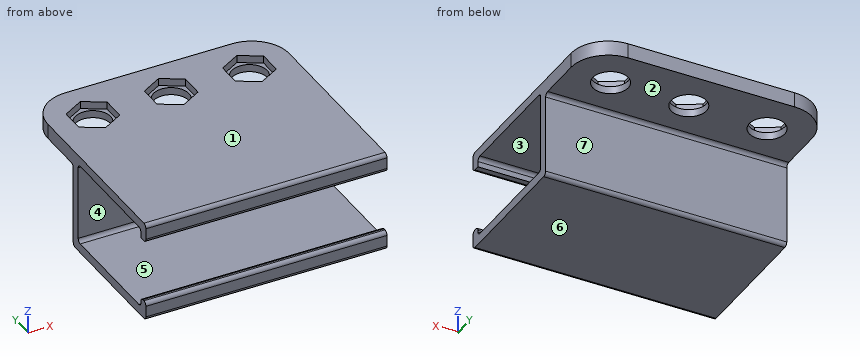
```python
from build123d import *

# Parameters (mm, degrees)
SKETCH_W     = 64.701706
SKETCH_H     = 22.701706
PAD_DEPTH    = 2
SKETCH001_W  = 64.701706
SKETCH001_H  = 22.701706
SKETCH001_R  = 4.75
PAD001_DEPTH = 2
PAD002_DEPTH = 64.701706
FILLET_R     = 10
FILLET001_R  = 1


with BuildPart() as part:
    # Sketch → Pad (new body)
    with BuildSketch(Plane.XY):
        Rectangle(SKETCH_W, SKETCH_H)
        Polygon((0, 6.350853), (-5.5, 3.175426), (-5.5, -3.175426), (0, -6.350853), (5.5, -3.175426), (5.5, 3.175426), align=None, mode=Mode.SUBTRACT)
        Polygon((-21, 6.350853), (-26.5, 3.175426), (-26.5, -3.175426), (-21, -6.350853), (-15.5, -3.175426), (-15.5, 3.175426), align=None, mode=Mode.SUBTRACT)
        Polygon((21, 6.350853), (15.5, 3.175426), (15.5, -3.175426), (21, -6.350853), (26.5, -3.175426), (26.5, 3.175426), align=None, mode=Mode.SUBTRACT)
    extrude(amount=PAD_DEPTH)

    # Sketch001 (on Face23 of Pad) → Pad001 (join)
    with BuildSketch(Plane(origin=(0, 0, 0), x_dir=(1, 0, 0), z_dir=(0, 0, -1))):
        Rectangle(SKETCH001_W, SKETCH001_H)
        Circle(SKETCH001_R, mode=Mode.SUBTRACT)
        with Locations((21, 0)):
            Circle(SKETCH001_R, mode=Mode.SUBTRACT)
        with Locations((-21, 0)):
            Circle(SKETCH001_R, mode=Mode.SUBTRACT)
    extrude(amount=PAD001_DEPTH)

    # Sketch002 (on Face28 of Pad001) → Pad002 (join)
    with BuildSketch(Plane(origin=(-32.350853, 0, 0), x_dir=(0, -1, 0), z_dir=(-1, 0, 0))):
        Polygon((11.350853, 2), (11.350853, -25), (47.850853, -25), (47.850853, -20), (45.350853, -20), (45.350853, -22.5), (13.850853, -22.5), (13.850853, -0.5), (45.350853, -0.5), (45.350853, -3), (47.850853, -3), (47.850853, 2), align=None)
    extrude(amount=-PAD002_DEPTH)

    # Fillet
    fillet_edges = [part.edges().sort_by_distance(p)[0] for p in [
        (32.350853, 11.350853, 0),
        (-32.350853, 11.350853, 0),
    ]]
    fillet(fillet_edges, radius=FILLET_R)

    # Fillet001
    fillet001_edges = [part.edges().sort_by_distance(p)[0] for p in [
        (0, -47.850853, 2),
        (0, -47.850853, -3),
        (0, -45.350853, -20),
        (0, -47.850853, -20),
        (0, -47.850853, -25),
        (0, -13.850853, -22.5),
        (0, -13.850853, -0.5),
        (0, -45.350853, -0.5),
        (0, -45.350853, -22.5),
        (0, -11.350853, -25),
        (0, -11.350853, -2),
    ]]
    fillet(fillet001_edges, radius=FILLET001_R)


solid = part.part
```
Work out the finished part from the listing and answer in its coordinate system (mm). Face numbers are marked on the shaded views. A direction names the side the tool comes from. Give positions to 0.01 mm unless a question says otherwise; leave off trailing zeros. Loops run counter-clockwise (first coordinate to the right, second up) from the corner with the lowest first, then second, coordinate; pieces in that order, holes last. Notation, with made-up numbers: (61.5, 82) -> (74.5, 82) arc R29 cw to (74.5, 117) -> close; hole circle Ø11 at (1.5, 29.25). An arc over 180 degrees is marked (long way). Use CSV: the item, a comma, the result in double quotes.
1. Straight lines are drawn through the part: line 1 (X direction, y = 0, z = -0.45); line 2 (Z direction, x = 5, y = -27.5); line 3 (Y direction, x = 0, z = -1). For each, find the intervals that lie inside material, in ascending order.
Found:
line 1,"-32.35 to -25.75, -16.25 to -4.75, 4.75 to 16.25, 25.75 to 32.35"
line 2,"-25 to -22.5, -0.5 to 2"
line 3,"-47.85 to -45.22, -13.98 to -4.75, 4.75 to 11.35"
2. A tool of negligible diameter and unlimited length cuts with its end or side. For the marked faces 5, 6 and 7, from which of +Z, -Z, +X, -X, +Y, -Y can it reach the whole face along a straight path? Write none if from no direction.
Found:
face 5,"+X, -X"
face 6,"-Z, +X, -X, +Y, -Y"
face 7,"-Z, +X, -X, +Y"
3. The part is cut by section A-A (y = -23). Write down the section's boundary in (x, z).
Found:
outline,"(-32.35, -25) -> (32.35, -25) -> (32.35, -22.5) -> (-32.35, -22.5) -> close; (-32.35, -0.5) -> (32.35, -0.5) -> (32.35, 2) -> (-32.35, 2) -> close"
4. The mould has two halves that part along Z. Classify the marked faces 1, 2, 3 and 4: +Z half, -Z half, draft (parallel to the pull), parting line (faces both ways), or undercut.
Found:
face 1,"+Z half"
face 2,"-Z half"
face 3,"undercut"
face 4,"undercut"
5. The part is cut by section C-C (x = 9.5). Write down the section's boundary in (y, z), then the cut area to 3 significant figures.
Found:
outline,"(-47.85, -24) arc R1 ccw to (-46.85, -25) -> (-12.35, -25) arc R1 ccw to (-11.35, -24) -> (-11.35, -3) arc R1 cw to (-10.35, -2) -> (11.35, -2) -> (11.35, 2) -> (-46.85, 2) arc R1 ccw to (-47.85, 1) -> (-47.85, -2) arc R1 ccw to (-46.85, -3) -> (-45.35, -3) -> (-45.35, -1.5) arc R1 cw to (-44.35, -0.5) -> (-14.85, -0.5) arc R1 cw to (-13.85, -1.5) -> (-13.85, -21.5) arc R1 cw to (-14.85, -22.5) -> (-44.35, -22.5) arc R1 cw to (-45.35, -21.5) -> (-45.35, -21) arc R1 ccw to (-46.35, -20) -> (-46.85, -20) arc R1 ccw to (-47.85, -21) -> close"
area,"341 mm^2"
6. Flat-ended cylindrical pins translate along their axes: pin 1 Ø12.5 at (x, y) = (21, 0) entering from -Z; pin 2 Ø1 at (x, z) = (23, -13.5) entering from +Y; pin 3 Ø6 at (x, z) = (10.5, -7) entering from -Y; pin 4 Ø5.5 at (x, y) = (-1.5, 2.5) entering from +Z. Find the tip coordinate at first contact, or state that the pin passes through.
Found:
pin 1,"z = -2"
pin 2,"y = -11.35"
pin 3,"y = -13.85"
pin 4,"z = 2"
7. The part is cut by section B-B (y = 0). Write down the section's boundary in (x, z), then the cut area to 3 significant figures.
Found:
outline,"(-32.35, -2) -> (-25.75, -2) -> (-25.75, 0) -> (-26.5, 0) -> (-26.5, 2) -> (-32.35, 2) -> close; (-16.25, -2) -> (-4.75, -2) -> (-4.75, 0) -> (-5.5, 0) -> (-5.5, 2) -> (-15.5, 2) -> (-15.5, 0) -> (-16.25, 0) -> close; (4.75, -2) -> (16.25, -2) -> (16.25, 0) -> (15.5, 0) -> (15.5, 2) -> (5.5, 2) -> (5.5, 0) -> (4.75, 0) -> close; (25.75, -2) -> (32.35, -2) -> (32.35, 2) -> (26.5, 2) -> (26.5, 0) -> (25.75, 0) -> close"
area,"136 mm^2"
